Geometry check sheet. Reference: the model listing, model coordinates, mm. Face numbers are marked on the shaded views. A direction names the side the tool comes from. Round coordinates to 2 decimals unless told otherwise and drop trailing zeros. Loops run counter-clockwise (first coordinate to the right, second up) from the corner with the lowest first, then second, coordinate; pieces in that order, holes last. Notation, with made-up numbers: (-26.5, 82.25) -> (-6.5, 82.25) arc R25 ccw to (-6.5, 112.25) -> close; hole circle Ø5 at (63, 7). An arc over 180 degrees is marked (long way). Use one line per item in the form item = value.
from build123d import *

# Parameters (mm, degrees)
BOSS_EXTRU_1_DEPTH = 4
BOSS_EXTRU_2_DEPTH = 4
BOSS_EXTRU_3_START = -4
BOSS_EXTRU_3_DEPTH = 4
CONG_1_R           = 30
CONG_2_R           = 30
CONG_3_R           = 10
BOSS_EXTRU_4_DEPTH = 4
BOSS_EXTRU_5_DEPTH = 4
ESQUISSE7_R        = 5
BOSS_EXTRU_6_DEPTH = 10
ESQUISSE9_R        = 5
BOSS_EXTRU_7_DEPTH = 14
CONG_4_R           = 10
CONG_5_R           = 3


with BuildPart() as part:
    # Esquisse1 → Boss.-Extru.1 (new body)
    with BuildSketch(Plane.XY):
        Polygon((-70, -110), (-66, -110), (-66, -156), (66, -156), (66, -110), (70, -110), (70, -156), (100, -156), (100, -160), (-100, -160), (-100, -156), (-70, -156), align=None)
    extrude(amount=-BOSS_EXTRU_1_DEPTH)

    # Esquisse2 → Boss.-Extru.2 (add)
    with BuildSketch(Plane(origin=(70, 0, 0), x_dir=(0, 0, -1), z_dir=(1, 0, 0))):
        with BuildLine():
            Line((0, -120), (-20, -100))
            ThreePointArc((-20, -100), (-27.071067812, -82.928932188), (-10, -90))
            Line((-10, -90), (4, -110))
            Line((4, -110), (0, -110))
            Line((0, -110), (0, -120))
        make_face()
    extrude(amount=-BOSS_EXTRU_2_DEPTH)

    # Esquisse3 → Boss.-Extru.3 (add)
    with BuildSketch(Plane.ZY.offset(70).offset(BOSS_EXTRU_3_START)):
        with BuildLine():
            Line((-4, -110), (10, -90))
            ThreePointArc((10, -90), (27.071067812, -82.928932188), (20, -100))
            Line((20, -100), (0, -120))
            Line((0, -120), (0, -110))
            Line((0, -110), (-4, -110))
        make_face()
    extrude(amount=BOSS_EXTRU_3_DEPTH)

    # Congé1
    cong_1_edges = [part.edges().sort_by_distance(p)[0] for p in [
        (68, -120, 0),
        (-68, -120, 0),
    ]]
    fillet(cong_1_edges, radius=CONG_1_R)

    # Congé2
    cong_2_edges = [part.edges().sort_by_distance(p)[0] for p in [
        (68, -110, -4),
        (-68, -110, -4),
    ]]
    fillet(cong_2_edges, radius=CONG_2_R)

    # Congé3
    cong_3_edges = [part.edges().sort_by_distance(p)[0] for p in [
        (-70, -156, -2),
        (-66, -156, -2),
        (66, -156, -2),
        (70, -156, -2),
    ]]
    fillet(cong_3_edges, radius=CONG_3_R)

    # Esquisse4 → Boss.-Extru.4 (add)
    with BuildSketch(Plane.ZY.offset(70)):
        Polygon((-4, -119.456666925), (-4, -100), (3, -100), align=None)
    extrude(amount=-BOSS_EXTRU_4_DEPTH)

    # Esquisse6 → Boss.-Extru.5 (add)
    with BuildSketch(Plane(origin=(70, 0, 0), x_dir=(0, 0, -1), z_dir=(1, 0, 0))):
        Polygon((4, -119.456666925), (4, -100), (-3, -100), align=None)
    extrude(amount=-BOSS_EXTRU_5_DEPTH)

    # Esquisse7 → Boss.-Extru.6 (add)
    with BuildSketch(Plane(origin=(70, 0, 0), x_dir=(0, 0, -1), z_dir=(1, 0, 0))):
        with Locations(Location((-20, -90, 0), (0, 0, 90))):
            Circle(ESQUISSE7_R)
    extrude(amount=BOSS_EXTRU_6_DEPTH)

    # Esquisse9 → Boss.-Extru.7 (add)
    with BuildSketch(Plane.ZY.offset(70)):
        with Locations(Location((20, -90, 0), (0, 0, 90))):
            Circle(ESQUISSE9_R)
    extrude(amount=-BOSS_EXTRU_7_DEPTH)

    # Congé4
    cong_4_edges = [part.edges().sort_by_distance(p)[0] for p in [
        (68, -100, 20),
        (68, -90, 10),
        (-68, -90, 10),
        (-68, -100, 20),
    ]]
    fillet(cong_4_edges, radius=CONG_4_R)

    # Congé5
    cong_5_edges = [part.edges().sort_by_distance(p)[0] for p in [
        (-68, -100, 3),
        (68, -100, 3),
    ]]
    fillet(cong_5_edges, radius=CONG_5_R)


solid = part.part
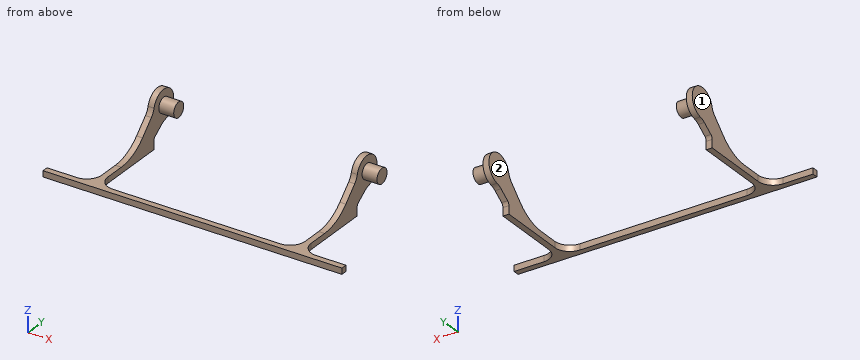
1. Section check B-B (z = 20). Record the boundary of the cut face in (x, y), then the cut area to 3 significant figures.
Return value:
outline = (-70, -100.61) -> (-66, -100.61) -> (-66, -95) -> (-56, -95) -> (-56, -85) -> (-66, -85) -> (-66, -80) -> (-70, -80) -> close; (66, -100.61) -> (70, -100.61) -> (70, -95) -> (80, -95) -> (80, -85) -> (70, -85) -> (70, -80) -> (66, -80) -> close
area = 365 mm2
2. Material ranges on line 1 along Y through (x, z) = (21, -2); line 2 along X through (y, z) = (-101, 11.5); line 3 along Z through (x, y) = (76.5, -90), recorded low to high.
Return value:
line_1 = -160 to -156
line_2 = -70 to -66, 66 to 70
line_3 = 15 to 25
3. Tool access check on the marked faces 1 and 2. Record the directions out of +Z, -Z, +X, -X, +Y, -Y that give a thin tool (end or side, any length) a straight path to the whole face; none if there is none.
Return value:
face_1 = +Z, -Z, -X, +Y
face_2 = +Z, -Z, +Y
4. Section check D-D (y = -114). Record the boundary of the cut face in (x, z).
Return value:
outline = (-70, -4) -> (-66, -4) -> (-66, 6.33) -> (-70, 6.33) -> close; (66, -4) -> (70, -4) -> (70, 6.33) -> (66, 6.33) -> close
5. Section check C-C (x = 42). Record the boundary of the cut face in (y, z), then the cut area to 3 significant figures.
Return value:
outline = (-160, -4) -> (-156, -4) -> (-156, 0) -> (-160, 0) -> close
area = 16.0 mm2
6. Section check A-A (y = -90). Record the boundary of the cut face in (x, z), then the cut area to 3 significant figures.
Return value:
outline = (-70, 9.65) -> (-66, 9.65) -> (-66, 15) -> (-56, 15) -> (-56, 25) -> (-66, 25) -> (-66, 30) -> (-70, 30) -> close; (66, 9.65) -> (70, 9.65) -> (70, 15) -> (80, 15) -> (80, 25) -> (70, 25) -> (70, 30) -> (66, 30) -> close
area = 363 mm2
7. Gauge pin test, flat ends, axial feed: pin 1 (14 mm diameter, centred on x = 18, y = -148, fed in from +Z); pin 2 (4.5 mm diameter, centred on x = 67.5, z = -2, fed in from +Y); pin 3 (4.5 mm diameter, centred on x = 91.5, z = -3, fed in from +Y); pin 4 (3 mm diameter, centred on y = -90, z = 17.5, fed in from +X). Record the tip position at first contact, or that the pin passes through.
Return value:
pin_1 = through
pin_2 = -100
pin_3 = -156
pin_4 = 80
